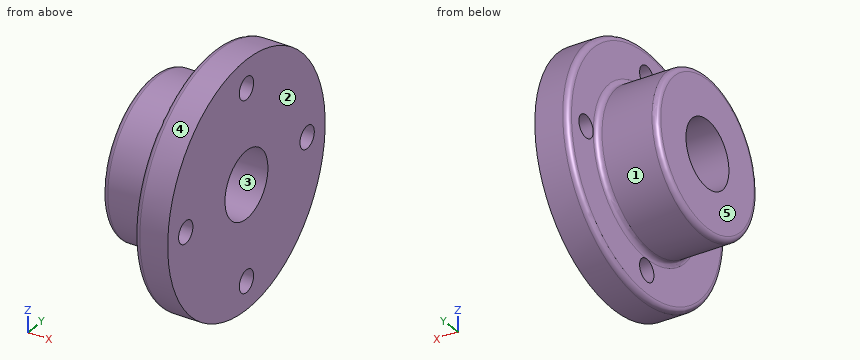
from build123d import *

# Parameters (mm, degrees)
F2_R     = 6.35
F3_DEPTH = 53.849
F4_R     = 3.04799
F5_R     = 3.048


# Not quite as in the source:
# - a fillet or chamfer is up to 0.001 mm smaller than in the source, because OpenCascade refuses the exact size


with BuildPart() as f1:
    # F0 (on Front) → F1 (revolve)
    with BuildSketch(Plane.XZ):
        Polygon((0, 44.45), (0, 19.05), (53.848, 19.05), (53.848, 69.85), (34.798, 69.85), (34.798, 44.45), align=None)
    revolve(axis=Axis((45.7144924702, 0, 0), (1, 0, 0)))

    # F2 (on Right) → F3 (cut, through all)
    with BuildSketch(Plane.YZ):
        with Locations((0, 53.848)):
            Circle(F2_R)
        with Locations((53.848, 0)):
            Circle(F2_R)
        with Locations((-53.848, 0)):
            Circle(F2_R)
        with Locations((0, -53.848)):
            Circle(F2_R)
    extrude(amount=F3_DEPTH, mode=Mode.SUBTRACT)

    # F4 (radius 3.048 in the source; OpenCascade refuses exactly that, so slightly less here)
    f4_edges = [f1.edges().sort_by_distance(p)[0] for p in [
        (34.798, 0, -44.45),
    ]]
    fillet(f4_edges, radius=F4_R)

    # F5
    f5_edges = [f1.edges().sort_by_distance(p)[0] for p in [
        (0, 0, -44.45),
        (34.798, 0, -69.85),
    ]]
    fillet(f5_edges, radius=F5_R)


solid = f1.part
Can you work these out from the model? Positions are in its coordinate system, mm. Face numbers are marked on the shaded views. A direction names the side the tool comes from. Round coordinates to 2 decimals unless told otherwise and drop trailing zeros. Order: outer loops, then holes, each group sorted by start corner. A loop starts at its lowest first (then second) coordinate and runs counter-clockwise, first axis right, second up. Notation, with made-up numbers: (86.25, -14.5) -> (136.25, -14.5) arc R24 cw to (136.25, 9.5) -> close; hole circle Ø11 at (11, 55.25). An arc over 180 degrees is marked (long way). Write each question's results on one line, items separated by ' | '. Start each with the question number.
Item 1: Thinking about a two-plate mould opening in Z: for the marked faces 3, 4 and 5, which applies, +Z half, -Z half, draft (parallel to the pull), parting line (faces both ways), or undercut?
Item 2: Please list where these lines run through material, in increasing order: L1, parallel to Z at x = 43, y = 0; L2, parallel to Y at x = 16, z = 0.
Item 3: If we section it at C-C, the plane x = 11.5: Write out the boundary of the cut face in (y, z).
Item 4: Which directions (+Z, -Z, +X, -X, +Y, -Y) give clear straight access to the entire face, cutting with the end or side of a thin tool? Please do the marked faces 1 and 2.
Item 5: If we section it at A-A, the plane y = 0: State how many separate pieces and enclosed holes the cut face has, then the cut area to 3 significant figures.
Item 6: Will these pins go through, and if not, where does the flat tip stop? pin 1 (3 mm diameter, centred on x = 19, y = 31.5, fed in from -Z); pin 2 (20.5 mm diameter, centred on y = 53.848, z = 0, fed in from -X); pin 3 (20.5 mm diameter, centred on y = -53.848, z = 0, fed in from +X); pin 4 (4 mm diameter, centred on x = 13.5, z = 2, fed in from +Y).
Results:
1) face 3: undercut | face 4: parting line | face 5: draft
2) L1: z = -69.85 to -60.2, -47.5 to -19.05, 19.05 to 47.5, 60.2 to 69.85 | L2: y = -44.45 to -19.05, 19.05 to 44.45
3) outline: circle Ø88.9 at (0, 0); hole circle Ø38.1 at (0, 0)
4) face 1: -X | face 2: +Z, -Z, +X, +Y, -Y
5) separate pieces: 4 | enclosed holes: 0 | area: 3,220 mm2
6) pin 1: stops at z = -32.8 | pin 2: stops at x = 0.93 | pin 3: stops at x = 53.85 | pin 4: stops at y = 44.45
